Here's how the part is built. I have some questions about the finished solid (model axes, mm). Coordinates: 2 decimals unless noted, no trailing zeros. Write each loop counter-clockwise with the first axis right and the second up, starting at its lowest first coordinate (ties: lowest second). Pieces come first, ordered by that corner, then holes.
Item 1: I'm going to push flat-ended pins straight in: P1, Ø1, axis at y = 18.5, z = 1, coming from the +X side; P2, Ø1.5, axis at y = 0, z = 2.5, coming from the +X side (3 decimals); P3, Ø10.5, axis at x = 0, y = -25, coming from the -Z side; P4, Ø2, axis at y = 13, z = 0.5, coming from the +X side. Where does each tip first touch, or does it pass through?
Item 2: If we mould it in two halves opening along X, with no side actions, what happens to faces 1 (the face through (-9.023, -40.635, 2.486)), 2 (the face through (-1.756, -7.907, 1.726)), 3 (the face through (13, -40, 1.5))? For each: pulls with the +X half, pulls with the -X half, needs draft (parallel to the pull), parting line crosses it, or undercut.
Item 3: I want a section at A-A (x = 0). Please give me the cut outline in (y, z) (3 decimals).
Item 4: I want a section at D-D (x = 24.5). Please give me the cut outline in (y, z).
Item 5: Please list where these lines run through material, in increasing order: line 1 (Y direction, x = -20, z = 1.4); line 2 (Y direction, x = 23, z = 1.8); line 3 (X direction, y = -12, z = 2.7).
Item 6: I want a section at C-C (z = 2.5). Please give me the cut outline in (x, y) (3 decimals).
Item 7: I want a section at B-B (y = 0). Please give me the cut outline in (x, z) (3 decimals).
from build123d import *

# Parameters (mm, degrees)
F0_R     = 41.625
F0_R_2   = 8.1
F1_DEPTH = 3.5
F0_R_3   = 45
F2_DEPTH = 1.5


with BuildPart() as f1:
    # F0 (on Top) → F1 (new body)
    with BuildSketch(Plane.XY):
        Circle(F0_R)
        with BuildLine():
            ThreePointArc((6.5, 25), (6.278518, 23.317676), (5.629165, 21.75))
            Line((5.629165, 21.75), (16.02147, 15.75))
            ThreePointArc((16.02147, 15.75), (23.332959, 18.778518), (28.150635, 12.5))
            ThreePointArc((28.150635, 12.5), (26.246829, 7.903806), (21.650635, 6))
            Line((21.650635, 6), (21.650635, -6))
            ThreePointArc((21.650635, -6), (26.246829, -7.903806), (28.150635, -12.5))
            ThreePointArc((28.150635, -12.5), (23.332959, -18.778518), (16.02147, -15.75))
            Line((16.02147, -15.75), (5.629165, -21.75))
            ThreePointArc((5.629165, -21.75), (6.278518, -23.317676), (6.5, -25))
            ThreePointArc((6.5, -25), (-1.682324, -31.278518), (-5.629165, -21.75))
            Line((-5.629165, -21.75), (-16.02147, -15.75))
            ThreePointArc((-16.02147, -15.75), (-27.2798, -15.75), (-21.650635, -6))
            Line((-21.650635, -6), (-21.650635, 6))
            ThreePointArc((-21.650635, 6), (-27.2798, 15.75), (-16.02147, 15.75))
            Line((-16.02147, 15.75), (-5.629165, 21.75))
            ThreePointArc((-5.629165, 21.75), (-1.682324, 31.278518), (6.5, 25))
        make_face(mode=Mode.SUBTRACT)
        with BuildLine():
            Line((16.02147, 15.75), (5.629165, 21.75))
            ThreePointArc((5.629165, 21.75), (0, 18.5), (-5.629165, 21.75))
            Line((-5.629165, 21.75), (-16.02147, 15.75))
            ThreePointArc((-16.02147, 15.75), (-15.372117, 14.182324), (-15.150635, 12.5))
            ThreePointArc((-15.150635, 12.5), (-17.054441, 7.903806), (-21.650635, 6))
            Line((-21.650635, 6), (-21.650635, -6))
            ThreePointArc((-21.650635, -6), (-17.054441, -7.903806), (-15.150635, -12.5))
            ThreePointArc((-15.150635, -12.5), (-15.372117, -14.182324), (-16.02147, -15.75))
            Line((-16.02147, -15.75), (-5.629165, -21.75))
            ThreePointArc((-5.629165, -21.75), (0, -18.5), (5.629165, -21.75))
            Line((5.629165, -21.75), (16.02147, -15.75))
            ThreePointArc((16.02147, -15.75), (16.02147, -9.25), (21.650635, -6))
            Line((21.650635, -6), (21.650635, 6))
            ThreePointArc((21.650635, 6), (16.02147, 9.25), (16.02147, 15.75))
        make_face()
        Circle(F0_R_2, mode=Mode.SUBTRACT)
    extrude(amount=F1_DEPTH)

    # F0 (on Top) → F2 (join)
    with BuildSketch(Plane.XY):
        Circle(F0_R_3)
        Circle(F0_R, mode=Mode.SUBTRACT)
    extrude(amount=F2_DEPTH)


solid = f1.part
Answer:
1. P1: stops at x = 41.24
1. P2: stops at x = 41.625
1. P3: passes through
1. P4: stops at x = 43.37
2. face 1: parting line crosses it
2. face 2: undercut
2. face 3: needs draft
3. outline: (-45, 0) - (-31.5, 0) - (-31.5, 3.5) - (-41.625, 3.5) - (-41.625, 1.5) - (-45, 1.5) - close; (-18.5, 0) - (-8.1, 0) - (-8.1, 3.5) - (-18.5, 3.5) - close; (8.1, 0) - (18.5, 0) - (18.5, 3.5) - (8.1, 3.5) - close; (31.5, 0) - (45, 0) - (45, 1.5) - (41.625, 1.5) - (41.625, 3.5) - (31.5, 3.5) - close
4. outline: (-37.75, 0) - (-18.34, 0) - (-18.34, 3.5) - (-33.65, 3.5) - (-33.65, 1.5) - (-37.75, 1.5) - close; (-6.66, 0) - (6.66, 0) - (6.66, 3.5) - (-6.66, 3.5) - close; (18.34, 0) - (37.75, 0) - (37.75, 1.5) - (33.65, 1.5) - (33.65, 3.5) - (18.34, 3.5) - close
5. line 1: y = -40.31 to -18.79, -6.21 to 6.21, 18.79 to 40.31
5. line 2: y = -34.69 to -18.86, -6.14 to 6.14, 18.86 to 34.69
5. line 3: x = -39.86 to -28.13, -15.17 to 15.17, 28.13 to 39.86
6. outline: circle Ø83.25 at (0, 0); hole (-16.021, -15.75) arc R6.5 ccw to (-15.151, -12.5) arc R6.5 ccw (long way) to start; hole (-16.021, 15.75) arc R6.5 ccw (long way) to (-15.151, 12.5) arc R6.5 ccw to start; hole circle Ø16.2 at (0, 0); hole (5.629, -21.75) arc R6.5 ccw (long way) to (6.5, -25) arc R6.5 ccw to start; hole (5.629, 21.75) arc R6.5 ccw to (6.5, 25) arc R6.5 ccw (long way) to start; hole circle Ø13 at (21.651, -12.5); hole circle Ø13 at (21.651, 12.5)
7. outline: (-45, 0) - (-8.1, 0) - (-8.1, 3.5) - (-41.625, 3.5) - (-41.625, 1.5) - (-45, 1.5) - close; (8.1, 0) - (45, 0) - (45, 1.5) - (41.625, 1.5) - (41.625, 3.5) - (8.1, 3.5) - close
